Verification items for the finished model (mm, model axes). A direction names the side the tool comes from. Give positions to 0.01 mm unless a question says otherwise; leave off trailing zeros. Write each loop counter-clockwise with the first axis right and the second up, starting at its lowest first coordinate (ties: lowest second). Pieces come first, ordered by that corner, then holes.
from build123d import *

# Parameters (mm, degrees)
CUT_EXTRUDE3_DEPTH      = 10
CUT_EXTRUDE3_DEPTH_BACK = 16
CUT_EXTRUDE4_DEPTH      = 16
SKETCH7_W               = 0.75
SKETCH7_H               = 1.5


with BuildPart() as part:
    # Sketch1 → Revolve1 (revolve)
    with BuildSketch(Plane(origin=(0, 0, 0), x_dir=(1, 0, 0), z_dir=(0, 1, 0)), mode=Mode.PRIVATE) as revolve1_sk:
        Polygon((4, 0), (10, 0), (10, 7), (11, 7), (11, 10), (15, 10), (15, 28), (14, 28), (14, 52), (11, 52), (11, 57), (10, 57), (10, 80), (4, 80), align=None)
    revolve(revolve1_sk.sketch.rotate(Axis((0, 0, -122.779357785), (0, 0, 1)), 180), axis=Axis((0, 0, -122.779357785), (0, 0, 1)))

    # Sketch5 → Cut-Extrude3 (cut, two sides: drawn at the far end of the back side and taken through both)
    with BuildSketch(Plane(origin=(0, 0, -52), x_dir=(-1, 0, 0), z_dir=(0, 0, -1)).offset(-CUT_EXTRUDE3_DEPTH_BACK)):
        Polygon((-4, 91.782839275), (-4, 13.416407865), (-4, 10), (4, 10), (4, 13.416407865), (4, 91.782839275), (4, 248.515702096), (-4, 248.515702096), align=None)
    extrude(amount=CUT_EXTRUDE3_DEPTH + CUT_EXTRUDE3_DEPTH_BACK, mode=Mode.SUBTRACT)

    # Sketch6 → Cut-Extrude4 (cut)
    with BuildSketch(Plane(origin=(0, 0, -80), x_dir=(-1, 0, 0), z_dir=(0, 0, -1))):
        Polygon((-3, 80.405860958), (-3, 9.539392014), (-3, 6.5), (3, 6.5), (3, 9.539392014), (3, 80.405860958), (3, 222.138798846), (-3, 222.138798846), align=None)
    extrude(amount=-CUT_EXTRUDE4_DEPTH, mode=Mode.SUBTRACT)

    # Sketch7 → Cut-Revolve1 (revolve, cut)
    with BuildSketch(Plane(origin=(0, 0, 0), x_dir=(1, 0, 0), z_dir=(0, 1, 0)), mode=Mode.PRIVATE) as cut_revolve1_sk:
        with Locations((9.625, 76.75)):
            Rectangle(SKETCH7_W, SKETCH7_H)
    revolve(cut_revolve1_sk.sketch.rotate(Axis((0, 0, 11.784239999), (0, 0, -1)), 252.542396876), axis=Axis((0, 0, 11.784239999), (0, 0, -1)), mode=Mode.SUBTRACT)


solid = part.part
Item 1: Depth check by flat-ended pin: pin 1 (8 mm diameter, centred on y = -12, z = -63.5, fed in from +X); pin 2 (2.5 mm diameter, centred on y = 12, z = -47.5, fed in from -X); pin 3 (3 mm diameter, centred on x = 5.5, z = -69, fed in from +Y); pin 4 (7 mm diameter, centred on x = 0, y = 0, fed in from -Z). Enter the tip coordinate at first touch or a pass-through.
Answer key:
pin 1: stops at x = 6
pin 2: stops at x = -8.97
pin 3: stops at y = 9.17
pin 4: passes through
Item 2: Scan lines: line 1 along Z through (x, y) = (8.25, -5); line 2 along Y through (x, z) = (0, -45); line 3 along Y through (x, z) = (0, -26). Record each from-to range of solid material in increasing order.
Answer key:
line 1: z = -80 to -77.5, -76 to 0
line 2: y = -14 to -4, 4 to 10
line 3: y = -15 to -4, 4 to 15
Item 3: Sectioned sample at B-B on z = -16. Record the cut outline in (x, y), then the cut area to 3 significant figures.
Answer key:
outline: circle Ø30 at (0, 0); hole circle Ø8 at (0, 0)
area: 657 mm2
Item 4: Set-up check for faces 1 (the face through (0, 10, -46)), 2 (the face through (-5.38, -8.43, -66.63)), 3 (the face through (4.3, -0.1, 0)), 4 (the face through (-5, -10, -10)), 5 (the face through (0.364, -9.243, -76.76)): record each of +Z, -Z, +X, -X, +Y, -Y from which the full face is reachable in a straight line by a thin tool's end or side.
Answer key:
face 1: -Z, +Y
face 2: -Z
face 3: +Z, +X, -X, +Y, -Y
face 4: +Z
face 5: none
Item 5: Sectioned sample at C-C on y = 12.25. Record the cut outline in (x, z).
Answer key:
outline: (-8.66, -28) - (-6.78, -28) - (-6.78, -52) - (-4, -52) - (-4, -36) - (4, -36) - (4, -52) - (6.78, -52) - (6.78, -28) - (8.66, -28) - (8.66, -10) - (-8.66, -10) - close
Item 6: Release check for a two-part mould opening along X. For faces 6 (the face through (10, 0, -4)), 7 (the face through (3, 8, -72)), 8 (the face through (-3, -9, -76)) record: released by +X, released by -X, zero draft, split by the parting line, or undercut.
Answer key:
face 6: split by the parting line
face 7: undercut
face 8: zero draft
